```python
from build123d import *

# Parameters (mm, degrees)
F0_R     = 11.303
F1_DEPTH = 7.239


# Not quite as in the source:
# - a feature names something its author has since deleted; it is built from what else it names


with BuildPart() as f1:
    # F0 (on Top) → F1 (new body)
    with BuildSketch(Plane.XY):
        with BuildLine():
            ThreePointArc((-5.8198711326, 12.7), (0, 13.97), (5.8198711326, 12.7))
            ThreePointArc((5.8198711326, 12.7), (8.1011295792, 14.0187610718), (10.0941728301, 15.7424343193))
            ThreePointArc((10.0941728301, 15.7424343193), (12.9648851602, 20.1968612567), (13.97, 25.4))
            ThreePointArc((13.97, 25.4), (-4.9295356548, 38.4713648189), (-10.4910706124, 16.1751239897))
            ThreePointArc((-10.4910706124, 16.1751239897), (-8.3385146662, 14.191517803), (-5.8198711326, 12.7))
        make_face()
        with Locations((0, 25.4)):
            Circle(F0_R, mode=Mode.SUBTRACT)
        with BuildLine():
            ThreePointArc((19.2536035907, 0.9979716684), (16.4594722687, 0.1256066293), (13.9084581944, -1.3098437524))
            ThreePointArc((13.9084581944, -1.3098437524), (12.0983748909, -6.985), (8.0885870618, -11.3901562476))
            ThreePointArc((8.0885870618, -11.3901562476), (8.0900384281, -14.0251645508), (8.5862616229, -16.6130272607))
            ThreePointArc((8.5862616229, -16.6130272607), (23.9734375051, -26.5294892776), (35.9670452561, -12.7))
            ThreePointArc((35.9670452561, -12.7), (30.852411424, -1.8952144846), (19.2536035907, 0.9979716684))
        make_face()
        with Locations((21.9970452561, -12.7)):
            Circle(F0_R, mode=Mode.SUBTRACT)
        with BuildLine():
            ThreePointArc((-8.0270452561, -12.7), (-8.042439189, -12.044355651), (-8.0885870618, -11.3901562476))
            ThreePointArc((-8.0885870618, -11.3901562476), (-12.0983748909, -6.985), (-13.9084581944, -1.3098437524))
            ThreePointArc((-13.9084581944, -1.3098437524), (-16.1911680073, 0.006403479), (-18.680434453, 0.8705929414))
            ThreePointArc((-18.680434453, 0.8705929414), (-34.2395365622, -19.4292129272), (-8.7625329783, -17.1730956581))
            ThreePointArc((-8.7625329783, -17.1730956581), (-8.2121434334, -14.9665793035), (-8.0270452561, -12.7))
        make_face()
        with Locations((-21.9970452561, -12.7)):
            Circle(F0_R, mode=Mode.SUBTRACT)
        with BuildLine():
            ThreePointArc((13.9084581944, -1.3098437524), (13.9546060671, -0.655644349), (13.97, 0))
            ThreePointArc((13.97, 0), (13.5166645575, 3.5299687308), (12.1860802806, 6.8308379717))
            ThreePointArc((12.1860802806, 6.8308379717), (9.4691782802, 10.2711032853), (5.8198711326, 12.7))
            ThreePointArc((5.8198711326, 12.7), (0, 11.43), (-5.8198711326, 12.7))
            ThreePointArc((-5.8198711326, 12.7), (-9.3380147919, 10.3904946824), (-12.0087193529, 7.1380361097))
            ThreePointArc((-12.0087193529, 7.1380361097), (-13.6296255101, 3.0649973009), (-13.9084581944, -1.3098437524))
            ThreePointArc((-13.9084581944, -1.3098437524), (-9.8986703653, -5.715), (-8.0885870618, -11.3901562476))
            ThreePointArc((-8.0885870618, -11.3901562476), (-4.3294249569, -13.2822053719), (-0.1773609276, -13.9688740814))
            ThreePointArc((-0.1773609276, -13.9688740814), (4.1604472299, -13.3361005863), (8.0885870618, -11.3901562476))
            ThreePointArc((8.0885870618, -11.3901562476), (9.8986703653, -5.715), (13.9084581944, -1.3098437524))
        make_face()
        Circle(F0_R, mode=Mode.SUBTRACT)
        with BuildLine():
            ThreePointArc((-13.9084581944, -1.3098437524), (-13.6296255101, 3.0649973009), (-12.0087193529, 7.1380361097))
            Line((-12.0087193529, 7.1380361097), (-18.680434453, 0.8705929414))
            ThreePointArc((-18.680434453, 0.8705929414), (-16.1911680073, 0.006403479), (-13.9084581944, -1.3098437524))
        make_face()
        with BuildLine():
            ThreePointArc((-12.0087193529, 7.1380361097), (-9.3380147919, 10.3904946824), (-5.8198711326, 12.7))
            ThreePointArc((-5.8198711326, 12.7), (-8.3385146662, 14.191517803), (-10.4910706124, 16.1751239897))
            Line((-10.4910706124, 16.1751239897), (-12.0087193529, 7.1380361097))
        make_face()
        with BuildLine():
            ThreePointArc((5.8198711326, 12.7), (9.4691782802, 10.2711032853), (12.1860802806, 6.8308379717))
            Line((12.1860802806, 6.8308379717), (10.0941728301, 15.7424343193))
            ThreePointArc((10.0941728301, 15.7424343193), (8.1011295792, 14.0187610718), (5.8198711326, 12.7))
        make_face()
        with BuildLine():
            ThreePointArc((12.1860802806, 6.8308379717), (13.5166645575, 3.5299687308), (13.97, 0))
            ThreePointArc((13.97, 0), (13.9546060671, -0.655644349), (13.9084581944, -1.3098437524))
            ThreePointArc((13.9084581944, -1.3098437524), (16.4594722687, 0.1256066293), (19.2536035907, 0.9979716684))
            Line((19.2536035907, 0.9979716684), (12.1860802806, 6.8308379717))
        make_face()
        with BuildLine():
            ThreePointArc((8.5862616229, -16.6130272607), (8.0900384281, -14.0251645508), (8.0885870618, -11.3901562476))
            ThreePointArc((8.0885870618, -11.3901562476), (4.1604472299, -13.3361005863), (-0.1773609276, -13.9688740814))
            Line((-0.1773609276, -13.9688740814), (8.5862616229, -16.6130272607))
        make_face()
        with BuildLine():
            Line((-8.7625329783, -17.1730956581), (-0.1773609276, -13.9688740814))
            ThreePointArc((-0.1773609276, -13.9688740814), (-4.3294249569, -13.2822053719), (-8.0885870618, -11.3901562476))
            ThreePointArc((-8.0885870618, -11.3901562476), (-8.042439189, -12.044355651), (-8.0270452561, -12.7))
            ThreePointArc((-8.0270452561, -12.7), (-8.2121434334, -14.9665793035), (-8.7625329783, -17.1730956581))
        make_face()
        with BuildLine():
            ThreePointArc((8.0885870618, -11.3901562476), (12.0983748909, -6.985), (13.9084581944, -1.3098437524))
            ThreePointArc((13.9084581944, -1.3098437524), (9.8986703653, -5.715), (8.0885870618, -11.3901562476))
        make_face()
        with BuildLine():
            ThreePointArc((-5.8198711326, 12.7), (0, 11.43), (5.8198711326, 12.7))
            ThreePointArc((5.8198711326, 12.7), (0, 13.97), (-5.8198711326, 12.7))
        make_face()
        with BuildLine():
            ThreePointArc((-13.9084581944, -1.3098437524), (-12.0983748909, -6.985), (-8.0885870618, -11.3901562476))
            ThreePointArc((-8.0885870618, -11.3901562476), (-9.8986703653, -5.715), (-13.9084581944, -1.3098437524))
        make_face()
    extrude(amount=F1_DEPTH)


solid = f1.part
```
Can you work these out from the model? Positions are in its coordinate system, mm. A direction names the side the tool comes from. Give positions to 0.01 mm unless a question says otherwise; leave off trailing zeros. Loops run counter-clockwise (first coordinate to the right, second up) from the corner with the lowest first, then second, coordinate; pieces in that order, holes last. Notation, with made-up numbers: M 89,42 L 144,42 A23 ccw 144,64 Z; hole C 84.25,85 d3. An arc over 180 degrees is marked long. One line per question, with ' | ' between items. Start each with the question number.
Q1. If we section it at C-C (z = 2.75): Please give me the cut outline in (x, y).
Q2. For faces 1 (the flat face through (-4.53, -15.593, 3.569)), 2 (the flat face through (-8.2, -8.2, 7.239)), which set-ups out of +Z, -Z, +X, -X, +Y, -Y let a thin tool reach every point of the face, with its end or its side?
Q3. For pin 1 Ø3 at (y, z) = (-4, 2) entering from -X; pin 2 Ø20.5 at (x, y) = (-22, -12.7) entering from -Z (3 decimals); pin 3 Ø2 at (x, z) = (-10, 1) entering from -Y; pin 4 Ø2 at (y, z) = (28, 2) entering from +X, each with a flat end and sliding along its axis, tell me the tip position at first contact or that it passes through.
Q4. If we section it at A-A (y = 8): Please give me the cut outline in (x, z).
Q5. If I drill on line 1 (Y direction, x = 0, z = 4); line 2 (X direction, y = -19.5, z = 6); line 3 (Y direction, x = -4, z = 5.25), over which ranges is the centre line in solid material (lowest first)? Write a range as from..to.
Q6. If we mould it in two halves opening along X, with no side actions, what happens to faces 3 (the flat face through (-11.24, 11.72, 3.57)), 4 (the flat face through (11.155, 11.224, 3.569)), 5 (the cylindrical face through (-34.45, -19.03, 3.57))? For each: +X half, -X half, draft (parallel to the pull), parting line (faces both ways), or undercut.
Q7. If we section it at B-B (x = -31): Please give me the cut outline in (y, z), plus the area to 3 significant figures.
Computed:
1) outline: M -18.68,0.87 A13.97 ccw long -8.76,-17.17 L -0.18,-13.97 L 8.59,-16.61 A13.97 ccw long 19.25,1 L 12.19,6.83 L 10.09,15.74 A13.97 ccw long -10.49,16.18 L -12.01,7.14 Z; hole C -22,-12.7 d22.61; hole C 0,0 d22.61; hole C 0,25.4 d22.61; hole C 22,-12.7 d22.61
2) face 1: +Z, -Z, -Y | face 2: +Z, +X, -X, +Y, -Y
3) pin 1: stops at x = -33.97 | pin 2: passes through | pin 3: stops at y = -21.32 | pin 4: stops at x = 13.88
4) outline: M -11.86,0 L -7.98,0 L -7.98,7.24 L -11.86,7.24 Z; M 7.98,0 L 11.91,0 L 11.91,7.24 L 7.98,7.24 Z
5) line 1: y = -14.02..-11.3, 11.3..14.1, 36.7..39.37 | line 2: x = -34.2..-31.03, -12.97..-9.79, 9.79..12.97, 31.03..34.2 | line 3: y = -15.4..-10.57, 10.57..14.83, 35.97..38.79
6) face 3: -X half | face 4: +X half | face 5: undercut
7) outline: M -23.38,0 L -19.53,0 L -19.53,7.24 L -23.38,7.24 Z; M -5.87,0 L -2.02,0 L -2.02,7.24 L -5.87,7.24 Z | area: 55.7 mm²
